For this review, take the finished solid that the model builds, in its own axes (mm). Face numbers are marked on the shaded views. A direction names the side the tool comes from. Round coordinates to 2 decimals unless told otherwise and drop trailing zeros. Loops run counter-clockwise (first coordinate to the right, second up) from the corner with the lowest first, then second, coordinate; pieces in that order, holes last.
1. To check wall thickness, follow line 1 along Y through (x, z) = (0.5, -4.5); line 2 along Z through (x, y) = (-19.5, 44); line 3 along Y through (x, z) = (-18.5, -5.25). State the ranges of each line that lie inside material, in increasing order.
2. Consider section D-D on y = -46.5. State the section outline as (x, z) points, then the cut area to 3 significant figures.
3. Consider section B-B on x = 0.5. State the section outline as (y, z) points, then the cut area to 4 significant figures.
4. Clearance check with flat-ended pins moving along their axes: pin 1 Ø1 at (x, y) = (8.5, 39) entering from -Z; pin 2 Ø2.5 at (x, z) = (8.5, -7.5) entering from +Y; pin 3 Ø2 at (y, z) = (10.5, -7) entering from +X. State where each tip first meets the part, or that it passes through.
5. Consider section C-C on z = -6.75. State the section outline as (x, y) points.
6. Consider section A-A on y = 26.2. State the section outline as (x, z) points, then the cut area to 4 significant figures.
7. Tool access review of the marked faces 1 and 2: name each direction out of +Z, -Z, +X, -X, +Y, -Y from which nothing blocks a thin tool from reaching the whole face with its end or side.
from build123d import *

# Parameters (mm, degrees)
F0_W     = 40
F0_H     = 100
F0_R     = 17.5
F0_R_2   = 1.45
F1_DEPTH = 5
F2_W     = 5
F2_H     = 100
F3_DEPTH = 10
F4_R     = 17.5
F4_R_2   = 16.5
F5_DEPTH = 1
F6_R     = 17.5
F6_R_2   = 16.5
F7_DEPTH = 1


with BuildPart() as f1:
    # F0 (on Top) → F1 (new body)
    with BuildSketch(Plane.XY):
        Rectangle(F0_W, F0_H)
        with Locations((0.5, 26.2)):
            Circle(F0_R, mode=Mode.SUBTRACT)
        with Locations((0.5, 26.2)):
            Circle(F0_R)
        with Locations((0.5, 26.2)):
            Circle(F0_R_2, mode=Mode.SUBTRACT)
    extrude(amount=-F1_DEPTH)

    # F2 (on face) → F3 (join)
    with BuildSketch(Plane.XY):
        with Locations((-22.5, 0)):
            Rectangle(F2_W, F2_H)
        Polygon((20, -50), (-20, -50), (-25, -50), (-25, -55), (20, -55), align=None)
    extrude(amount=-F3_DEPTH)

    # F4 (on face) → F5 (cut)
    with BuildSketch(Plane.XY):
        with Locations((0.5, 26.2)):
            Circle(F4_R)
        with Locations((0.5, 26.2)):
            Circle(F4_R_2, mode=Mode.SUBTRACT)
    extrude(amount=-F5_DEPTH, mode=Mode.SUBTRACT)

    # F6 (on face) → F7 (cut)
    with BuildSketch(Plane(origin=(0, 0, -5), x_dir=(1, 0, 0), z_dir=(0, 0, -1))):
        with Locations((0.5, -26.2)):
            Circle(F6_R)
        with Locations((0.5, -26.2)):
            Circle(F6_R_2, mode=Mode.SUBTRACT)
    extrude(amount=-F7_DEPTH, mode=Mode.SUBTRACT)


solid = f1.part
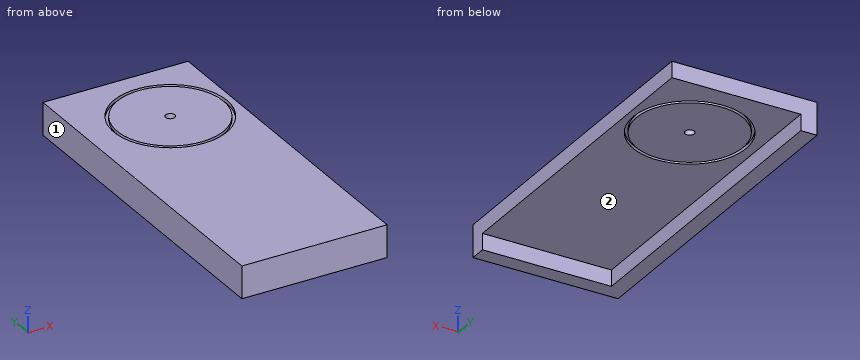
Resolved:
1. line 1: y = -55 to 8.7, 9.7 to 24.75, 27.65 to 42.7, 43.7 to 50
1. line 2: z = -5 to 0
1. line 3: y = -55 to -50
2. outline: (-25, -10) - (-20, -10) - (-20, -5) - (20, -5) - (20, 0) - (-25, 0) - close
2. area: 250 mm2
3. outline: (-55, -10) - (-50, -10) - (-50, -5) - (8.7, -5) - (8.7, -4) - (9.7, -4) - (9.7, -5) - (24.75, -5) - (24.75, 0) - (9.7, 0) - (9.7, -1) - (8.7, -1) - (8.7, 0) - (-55, 0) - close; (27.65, -5) - (42.7, -5) - (42.7, -4) - (43.7, -4) - (43.7, -5) - (50, -5) - (50, 0) - (43.7, 0) - (43.7, -1) - (42.7, -1) - (42.7, 0) - (27.65, 0) - close
3. area: 531.5 mm2
4. pin 1: stops at z = -5
4. pin 2: stops at y = -50
4. pin 3: stops at x = -20
5. outline: (-25, -55) - (20, -55) - (20, -50) - (-20, -50) - (-20, 50) - (-25, 50) - close
6. outline: (-25, -10) - (-20, -10) - (-20, -5) - (-17, -5) - (-17, -4) - (-16, -4) - (-16, -5) - (-0.95, -5) - (-0.95, 0) - (-16, 0) - (-16, -1) - (-17, -1) - (-17, 0) - (-25, 0) - close; (1.95, -5) - (17, -5) - (17, -4) - (18, -4) - (18, -5) - (20, -5) - (20, 0) - (18, 0) - (18, -1) - (17, -1) - (17, 0) - (1.95, 0) - close
6. area: 231.5 mm2
7. face 1: +Z, -Z, -X, +Y, -Y
7. face 2: -Z, +X, +Y
